The model under review builds one solid part; all positions refer to its coordinate system, in mm. Face numbers are marked on the shaded views. A direction names the side the tool comes from. Coordinates: 2 decimals unless noted, no trailing zeros. Write each loop counter-clockwise with the first axis right and the second up, starting at its lowest first coordinate (ties: lowest second). Pieces come first, ordered by that corner, then holes. Notation, with made-up numbers: (30, 33.25) - (64, 33.25) arc R17 ccw to (64, 59.25) - close; hole circle Ø5 at (73, 68). An arc over 180 degrees is marked (long way). Put each result on its own line as item: value.
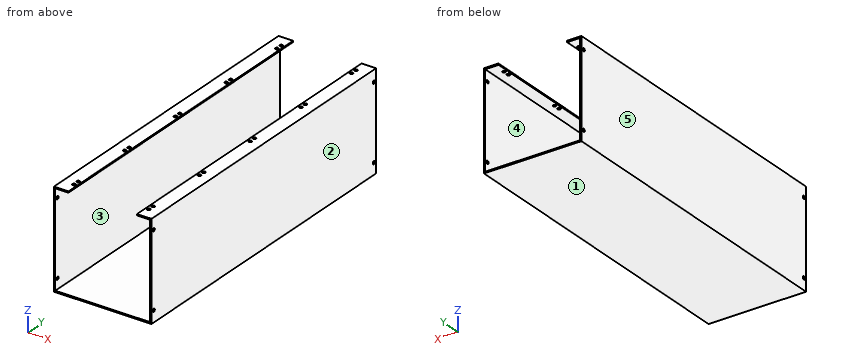
from build123d import *

# Parameters (mm, degrees)
BOSS_EXTRUDE1_DEPTH = 327.5
SKETCH2_R           = 1.6
CUT_EXTRUDE1_DEPTH  = 1.3
SKETCH4_R           = 1.6
CUT_EXTRUDE2_DEPTH  = 100


with BuildPart() as part:
    # Sketch1 → Boss-Extrude1 (new body)
    with BuildSketch(Plane(origin=(0, 0, 0), x_dir=(1, 0, 0), z_dir=(0, 1, 0))):
        Polygon((0, 0), (14.9, 0), (14.9, 1.3), (1.3, 1.3), (1.3, 98.7), (98.7, 98.7), (98.7, 1.3), (85.1, 1.3), (85.1, 0), (100, 0), (100, 100), (0, 100), align=None)
    extrude(amount=BOSS_EXTRUDE1_DEPTH)

    # Sketch2 → Cut-Extrude1 (cut)
    with BuildSketch(Plane.XY):
        with Locations((11.7, 314.9)):
            Circle(SKETCH2_R)
        with Locations((11.7, 308.5)):
            Circle(SKETCH2_R)
        with Locations((11.7, 240.925)):
            Circle(SKETCH2_R)
        with Locations((11.7, 234.525)):
            Circle(SKETCH2_R)
        with Locations((11.7, 166.95)):
            Circle(SKETCH2_R)
        with Locations((11.7, 160.55)):
            Circle(SKETCH2_R)
        with Locations((11.7, 92.975)):
            Circle(SKETCH2_R)
        with Locations((11.7, 86.575)):
            Circle(SKETCH2_R)
        with Locations((11.7, 19)):
            Circle(SKETCH2_R)
        with Locations((11.7, 12.6)):
            Circle(SKETCH2_R)
        with Locations((88.3, 314.9)):
            Circle(SKETCH2_R)
        with Locations((88.3, 308.5)):
            Circle(SKETCH2_R)
        with Locations((88.3, 240.925)):
            Circle(SKETCH2_R)
        with Locations((88.3, 234.525)):
            Circle(SKETCH2_R)
        with Locations((88.3, 166.95)):
            Circle(SKETCH2_R)
        with Locations((88.3, 160.55)):
            Circle(SKETCH2_R)
        with Locations((88.3, 19)):
            Circle(SKETCH2_R)
        with Locations((88.3, 12.6)):
            Circle(SKETCH2_R)
        with Locations((88.3, 86.575)):
            Circle(SKETCH2_R)
        with Locations((88.3, 92.975)):
            Circle(SKETCH2_R)
    extrude(amount=-CUT_EXTRUDE1_DEPTH, mode=Mode.SUBTRACT)

    # Sketch4 → Cut-Extrude2 (cut)
    with BuildSketch(Plane.ZY):
        with Locations((-88.3, 324.3)):
            Circle(SKETCH4_R)
        with Locations((-11.7, 324.3)):
            Circle(SKETCH4_R)
        with Locations((-88.3, 3.2)):
            Circle(SKETCH4_R)
        with Locations((-11.7, 3.2)):
            Circle(SKETCH4_R)
    extrude(amount=-CUT_EXTRUDE2_DEPTH, mode=Mode.SUBTRACT)


solid = part.part
1. For pin 1 Ø1 at (x, y) = (49.5, 292) entering from +Z; pin 2 Ø1.9 at (y, z) = (3.2, -11.7) entering from +X, all flat-tipped, find the tip position at first contact; note any pin that passes through.
Determined:
pin 1: stops at z = -98.7
pin 2: passes through
2. Consider section C-C on y = 113.5. State the section outline as (x, z) points, plus the area to 3 significant figures.
Determined:
outline: (0, -100) - (100, -100) - (100, 0) - (85.1, 0) - (85.1, -1.3) - (98.7, -1.3) - (98.7, -98.7) - (1.3, -98.7) - (1.3, -1.3) - (14.9, -1.3) - (14.9, 0) - (0, 0) - close
area: 422 mm^2
3. To check wall thickness, follow probe 1 along X at (y, z) = (160.55, -0.4); probe 2 along Y at (x, z) = (99.15, -11.7); probe 3 along X at (y, z) = (256, -72.5). State the ranges of each line that lie inside material, in increasing order.
Determined:
probe 1: x = 0 to 10.1, 13.3 to 14.9, 85.1 to 86.7, 89.9 to 100
probe 2: y = 0 to 1.6, 4.8 to 322.7, 325.9 to 327.5
probe 3: x = 0 to 1.3, 98.7 to 100
4. Consider section D-D on x = 54.5. State the section outline as (y, z) points, plus the area to 3 significant figures.
Determined:
outline: (0, -100) - (327.5, -100) - (327.5, -98.7) - (0, -98.7) - close
area: 426 mm^2
5. The part is to be moulded in two halves that separate along Z. For the marked faces 1, 2 and 3, say which applies: +Z half, -Z half, draft (parallel to the pull), parting line (faces both ways), or undercut.
Determined:
face 1: -Z half
face 2: draft
face 3: undercut
6. Machinability: for the marked faces 4 and 5, which of the approach directions +Z, -Z, +X, -X, +Y, -Y give a long, thin tool a straight path to every point of the face, cutting with its end or side? Answer none if there is none.
Determined:
face 4: +Y, -Y
face 5: +Z, -Z, -X, +Y, -Y
7. Consider section B-B on z = -29.5. State the section outline as (x, y) points.
Determined:
outline: (0, 0) - (1.3, 0) - (1.3, 327.5) - (0, 327.5) - close; (98.7, 0) - (100, 0) - (100, 327.5) - (98.7, 327.5) - close
8. Consider section A-A on x = 6. State the section outline as (y, z) points, plus the area to 4 significant figures.
Determined:
outline: (0, -100) - (327.5, -100) - (327.5, -98.7) - (0, -98.7) - close; (0, -1.3) - (327.5, -1.3) - (327.5, 0) - (0, 0) - close
area: 851.5 mm^2
